```python
from build123d import *

# Parameters (mm, degrees)
F0_W     = 100
F0_H     = 55
F1_DEPTH = 25
F3_DEPTH = 100
F5_DEPTH = 19
F7_D     = 5
F7_DEPTH = 8
F7_TIP   = 1.5021515476
F9_D     = 5
F9_DEPTH = 8
F9_TIP   = 1.5021515476


with BuildPart() as f1:
    # F0 (on Top) → F1 (new body)
    with BuildSketch(Plane.XY):
        Rectangle(F0_W, F0_H)
    extrude(amount=F1_DEPTH)

    # F2 (on face) → F3 (cut, through all)
    with BuildSketch(Plane.YZ.offset(50)):
        Polygon((15.5, 25), (-15.5, 25), (-18.5, 19), (18.5, 19), align=None)
    extrude(amount=-F3_DEPTH, mode=Mode.SUBTRACT)

    # F4 (on face) → F5 (cut, through all)
    with BuildSketch(Plane.XY.offset(19)):
        with BuildLine():
            Line((35, 14), (-35, 14))
            ThreePointArc((-35, 14), (-38.5355339059, 12.5355339059), (-40, 9))
            Line((-40, 9), (-40, -9))
            ThreePointArc((-40, -9), (-38.5355339059, -12.5355339059), (-35, -14))
            Line((-35, -14), (35, -14))
            ThreePointArc((35, -14), (38.5355339059, -12.5355339059), (40, -9))
            Line((40, -9), (40, 9))
            ThreePointArc((40, 9), (38.5355339059, 12.5355339059), (35, 14))
        make_face()
    extrude(amount=-F5_DEPTH, mode=Mode.SUBTRACT)

    # F7
    with Locations(Plane.YZ.offset(50)):
        with Locations((19.5, 8), (0, 8), (-19.5, 8)):
            Hole(F7_D / 2, depth=F7_DEPTH)
            with Locations((0, 0, -(F7_DEPTH + F7_TIP / 2))):  # 118° drill point
                Cone(0, F7_D / 2, F7_TIP, mode=Mode.SUBTRACT)

    # F9
    with Locations(Plane(origin=(-50, 0, 0), x_dir=(0, -1, 0), z_dir=(-1, 0, 0))):
        with Locations((-19.5, 8), (0, 8), (19.5, 8)):
            Hole(F9_D / 2, depth=F9_DEPTH)
            with Locations((0, 0, -(F9_DEPTH + F9_TIP / 2))):  # 118° drill point
                Cone(0, F9_D / 2, F9_TIP, mode=Mode.SUBTRACT)


solid = f1.part
```
Source: CAD feature listing. Evaluate the final solid. Frame: model axes, mm. A direction names the side the tool comes from. Round coordinates to 2 decimals unless told otherwise and drop trailing zeros. Loops run counter-clockwise (first coordinate to the right, second up) from the corner with the lowest first, then second, coordinate; pieces in that order, holes last.
1. Section query C-C on z = 12.5. Output: boundary loops of the cut face in (x, y), and give its area (3 significant figures).
2. Mould query, pull axis X, two halves, no side actions, for faces 1 (the flat face through (40, 0, 10)), 2 (the cylindrical face through (46, -18, 6)), 3 (the flat face through (-40, 0, 10)), 4 (the conical face through (40.76, 19.73, 8.37)). Classes: released by +X, released by -X, zero draft, split by the parting line, or undercut.
3. Contact query for flat-ended pins moving along their axis: pin 1 (3 mm diameter, centred on y = 19.5, z = 8, fed in from -X); pin 2 (4 mm diameter, centred on y = 0, z = 8, fed in from +X); pin 3 (4 mm diameter, centred on y = 19.5, z = 8, fed in from -X). Output: stop coordinate, or through.
4. Ray query, L1, parallel to Y at x = 46.5, z = 8; L2, parallel to Z at x = -45.25, y = -19.5; L3, parallel to X at y = -7, z = 16. Return the intervals inside material, ascending.
5. Section query A-A on x = -15. Output: boundary loops of the cut face in (y, z), and give its area (3 significant figures).
6. Section query D-D on y = 12. Output: boundary loops of the cut face in (x, z).
7. Section query B-B on y = -3.5. Output: boundary loops of the cut face in (x, z).
8. Access query for faces 5 (the flat face through (-1, 22, 25)), 6 (the flat face through (0, 14, 10)), 7 (the cylindrical face through (-45.94, -0.54, 5.56)), 8 (the flat face through (1, -17, 19)), 9 (the cylindrical face through (45.94, 0.54, 5.56)). Directions: +Z, -Z, +X, -X, +Y, -Y. A direction counts if a zero-diameter tool reaches every point of the face in a straight line with its end or side. Return the directions, or none.
Answers below:
1. outline: (-50, -27.5) - (50, -27.5) - (50, 27.5) - (-50, 27.5) - close; hole (-40, -9) arc R5 ccw to (-35, -14) - (35, -14) arc R5 ccw to (40, -9) - (40, 9) arc R5 ccw to (35, 14) - (-35, 14) arc R5 ccw to (-40, 9) - close
1. area: 3,280 mm2
2. face 1: undercut
2. face 2: zero draft
2. face 3: undercut
2. face 4: released by +X
3. pin 1: stops at x = -41.4
3. pin 2: stops at x = 41.7
3. pin 3: stops at x = -41.7
4. L1: y = -27.5 to -22, -17 to -2.5, 2.5 to 17, 22 to 27.5
4. L2: z = 0 to 5.5, 10.5 to 25
4. L3: x = -50 to -40, 40 to 50
5. outline: (-27.5, 0) - (-14, 0) - (-14, 19) - (-18.5, 19) - (-15.5, 25) - (-27.5, 25) - close; (14, 0) - (27.5, 0) - (27.5, 25) - (15.5, 25) - (18.5, 19) - (14, 19) - close
5. area: 639 mm2
6. outline: (-50, 0) - (-39, 0) - (-39, 19) - (-50, 19) - close; (39, 0) - (50, 0) - (50, 19) - (39, 19) - close
7. outline: (-50, 0) - (-40, 0) - (-40, 19) - (-50, 19) - close; (40, 0) - (50, 0) - (50, 19) - (40, 19) - close
8. face 5: +Z, +X, -X, +Y, -Y
8. face 6: +Z, -Z
8. face 7: -X
8. face 8: +X, -X
8. face 9: +X
